from build123d import *

# Parameters (mm, degrees)
SKETCH1_W           = 139.7
SKETCH1_H           = 63.5
BOSS_EXTRUDE1_DEPTH = 8.89
SKETCH2_R           = 1.4
CUT_EXTRUDE1_DEPTH  = 16.51
BOSS_EXTRUDE2_DEPTH = 8.89
FILLET1_R           = 10.16
FILLET2_R           = 5.08
FILLET3_R           = 43.18
SKETCH4_R           = 1.5
SKETCH4_R_2         = 2.5
CUT_EXTRUDE3_DEPTH  = 11.43
CUT_EXTRUDE6_DEPTH  = 198.882
SKETCH22_R          = 2.75
CUT_EXTRUDE8_DEPTH  = 4.572
SKETCH23_R          = 2.75
CUT_EXTRUDE9_DEPTH  = 4.572


with BuildPart() as part:
    # Sketch1 → Boss-Extrude1 (new body)
    with BuildSketch(Plane(origin=(0, 0, 0), x_dir=(1, 0, 0), z_dir=(0, 1, 0))):
        with Locations((69.85, 31.75)):
            Rectangle(SKETCH1_W, SKETCH1_H)
    extrude(amount=BOSS_EXTRUDE1_DEPTH)

    # Sketch2 → Cut-Extrude1 (cut)
    with BuildSketch(Plane(origin=(0, 8.89, 0), x_dir=(1, 0, 0), z_dir=(0, 1, 0))):
        with Locations((69.85, 60.325)):
            Circle(SKETCH2_R)
        with Locations((69.85, 3.175)):
            Circle(SKETCH2_R)
        with Locations((90.17, 3.175)):
            Circle(SKETCH2_R)
        with Locations((110.49, 3.175)):
            Circle(SKETCH2_R)
        with Locations((130.81, 3.175)):
            Circle(SKETCH2_R)
        with Locations((49.53, 3.175)):
            Circle(SKETCH2_R)
        with Locations((29.21, 3.175)):
            Circle(SKETCH2_R)
        with Locations((8.89, 3.175)):
            Circle(SKETCH2_R)
        with Locations((90.17, 60.325)):
            Circle(SKETCH2_R)
        with Locations((110.49, 60.325)):
            Circle(SKETCH2_R)
        with Locations((130.81, 60.325)):
            Circle(SKETCH2_R)
        with Locations((49.53, 60.325)):
            Circle(SKETCH2_R)
        with Locations((29.21, 60.325)):
            Circle(SKETCH2_R)
        with Locations((8.89, 60.325)):
            Circle(SKETCH2_R)
    extrude(amount=-CUT_EXTRUDE1_DEPTH, mode=Mode.SUBTRACT)


with BuildPart() as body_2:
    # Sketch3 → Boss-Extrude2 (new body)
    with BuildSketch(Plane(origin=(0, 8.89, 0), x_dir=(1, 0, 0), z_dir=(0, 1, 0))):
        with BuildLine():
            ThreePointArc((83.917692308, 197.377538462), (69.85, 206.756), (55.782307692, 197.377538462))
            Line((55.782307692, 197.377538462), (0, 63.5))
            Line((0, 63.5), (31.75, 63.5))
            Line((31.75, 63.5), (69.85, 154.94))
            Line((69.85, 154.94), (107.95, 63.5))
            Line((107.95, 63.5), (139.7, 63.5))
            Line((139.7, 63.5), (83.917692308, 197.377538462))
        make_face()
    extrude(amount=-BOSS_EXTRUDE2_DEPTH)

    # Fillet1
    fillet1_edges = [body_2.edges().sort_by_distance(p)[0] for p in [
        (69.85, 4.445, -154.94),
    ]]
    fillet(fillet1_edges, radius=FILLET1_R)


with BuildPart() as part_1:
    add(part.part)

    # Combine1: union body 2
    add(body_2.part)

    # Fillet2
    fillet2_edges = [part_1.edges().sort_by_distance(p)[0] for p in [
        (31.75, 4.445, -63.5),
        (107.95, 4.445, -63.5),
    ]]
    fillet(fillet2_edges, radius=FILLET2_R)

    # Fillet3
    fillet3_edges = [part_1.edges().sort_by_distance(p)[0] for p in [
        (0, 4.445, -63.5),
        (139.7, 4.445, -63.5),
    ]]
    fillet(fillet3_edges, radius=FILLET3_R)

    # Sketch4 → Cut-Extrude3 (cut)
    with BuildSketch(Plane(origin=(0, 8.89, 0), x_dir=(1, 0, 0), z_dir=(0, 1, 0))):
        with Locations((81.51726189, 192.00726189)):
            Circle(SKETCH4_R)
        with Locations((81.51726189, 168.67273811)):
            Circle(SKETCH4_R)
        with Locations((58.18273811, 192.00726189)):
            Circle(SKETCH4_R)
        with Locations((58.18273811, 168.67273811)):
            Circle(SKETCH4_R)
        with Locations((69.85, 180.34)):
            Circle(SKETCH4_R_2)
    extrude(amount=-CUT_EXTRUDE3_DEPTH, mode=Mode.SUBTRACT)

    # Sketch20 → Cut-Extrude6 (cut)
    with BuildSketch(Plane.ZY):
        Polygon((-206.756, 8.89), (-54.864, 8.89), (-206.756, 4.445), align=None)
        Polygon((-54.864, 8.89), (0, 3.81), (0, 8.89), align=None)
    extrude(amount=-CUT_EXTRUDE6_DEPTH, mode=Mode.SUBTRACT)

    # Sketch22 → Cut-Extrude8 (cut)
    with BuildSketch(Plane(origin=(0, 10.4865712, -0.306881264), x_dir=(1, 0, 0), z_dir=(0, 0.999572078, -0.029251691))):
        with Locations((130.81, 60.043812821)):
            Circle(SKETCH22_R)
        with Locations((110.49, 60.043812821)):
            Circle(SKETCH22_R)
        with Locations((90.17, 60.043812821)):
            Circle(SKETCH22_R)
        with Locations((69.85, 60.043812821)):
            Circle(SKETCH22_R)
        with Locations((49.53, 60.043812821)):
            Circle(SKETCH22_R)
        with Locations((29.21, 60.043812821)):
            Circle(SKETCH22_R)
        with Locations((8.89, 60.043812821)):
            Circle(SKETCH22_R)
    extrude(amount=-CUT_EXTRUDE8_DEPTH, mode=Mode.SUBTRACT)

    # Sketch23 → Cut-Extrude9 (cut)
    with BuildSketch(Plane(origin=(0, 3.81, 0), x_dir=(-1, 0, 0), z_dir=(0, -1, 0))):
        with Locations((-8.89, 3.175)):
            Circle(SKETCH23_R)
        with Locations((-29.21, 3.175)):
            Circle(SKETCH23_R)
        with Locations((-49.53, 3.175)):
            Circle(SKETCH23_R)
        with Locations((-69.85, 3.175)):
            Circle(SKETCH23_R)
        with Locations((-90.17, 3.175)):
            Circle(SKETCH23_R)
        with Locations((-110.49, 3.175)):
            Circle(SKETCH23_R)
        with Locations((-130.81, 3.175)):
            Circle(SKETCH23_R)
    extrude(amount=-CUT_EXTRUDE9_DEPTH, mode=Mode.SUBTRACT)


solid = part_1.part
Here's how the part is built. I have some questions about the finished solid (model axes, mm). A direction names the side the tool comes from. Coordinates: 2 decimals unless noted, no trailing zeros. Loops run counter-clockwise (first coordinate to the right, second up) from the corner with the lowest first, then second, coordinate; pieces in that order, holes last.
1. I need wall thicknesses on L1, parallel to Z at x = 49.53, y = 4 (3 decimals); L2, parallel to Y at x = 101.5, z = -11.5; L3, parallel to Z at x = 131, y = 3.25. Which ranges of each line are inside material? Lowest first, please.
2. For P1, Ø3.5, axis at x = 8.89, z = -3.175, coming from the +Y side; P2, Ø4, axis at x = 113, y = 2, coming from the -Z side; P3, Ø4.5, axis at x = 84.5, y = 5.5, coming from the -Z side, each with a flat end and sliding along its axis, tell me the tip position at first contact or that it passes through.
3. Imagine slicing it at B-B, the plane y = 2. Count the separate pieces of the cut face and the enclosed holes in it, and give its area (3 significant figures).
4. Imagine slicing it at C-C, the plane z = -38.5. Please give me the cut outline in (x, y), and give its area (3 significant figures).
5. For faces 1 (the cylindrical face through (69.683, 3.264, -138.683)), 2 (the flat face through (29.92, 3.33, -135.31)), 3 (the cylindrical face through (110.85, 4.03, -5.9)), which set-ups out of +Z, -Z, +X, -X, +Y, -Y let a thin tool reach every point of the face, with its end or its side?
6. Imagine slicing it at D-D, the plane z = -145. Please give me the cut outline in (x, y), and give its area (3 significant figures).
7. Imagine slicing it at A-A, the plane z = -80.5. Please give me the cut outline in (x, y), and give its area (3 significant figures).
Taken from the geometry:
1. L1: z = -182.372 to -106.172, -63.5 to -61.725, -58.925 to -5.925
1. L2: y = 0 to 4.87
1. L3: z = -84.38 to -61.71, -58.94 to -4.56, -1.79 to 0
2. P1: stops at y = 3.81
2. P2: stops at z = -132.38
2. P3: stops at z = -200.13
3. separate pieces: 1
3. enclosed holes: 20
3. area: 16,800 mm2
4. outline: (0, 0) - (139.7, 0) - (139.7, 7.37) - (0, 7.37) - close
4. area: 1,030 mm2
5. face 1: +Y, -Y
5. face 2: -Z, -X, +Y, -Y
5. face 3: +Y
6. outline: (33.96, 0) - (105.74, 0) - (105.74, 6.25) - (33.96, 6.25) - close
6. area: 449 mm2
7. outline: (7.08, 0) - (38.83, 0) - (38.83, 8.14) - (7.08, 8.14) - close; (100.87, 0) - (132.62, 0) - (132.62, 8.14) - (100.87, 8.14) - close
7. area: 517 mm2
